Geometry check sheet. Reference: the model listing, model coordinates, mm. Face numbers are marked on the shaded views. A direction names the side the tool comes from. Give positions to 0.01 mm unless a question says otherwise; leave off trailing zeros. Loops run counter-clockwise (first coordinate to the right, second up) from the corner with the lowest first, then second, coordinate; pieces in that order, holes last.
Autodesk Inventor part; units mm, degrees
ref_plane "YZ Plane" through (0, 0, 0) normal (1, 0, 0) x (0, 1, 0)
ref_plane "XZ Plane" through (0, 0, 0) normal (0, 1, 0) x (-1, 0, 0)
ref_plane "XY Plane" through (0, 0, 0) normal (0, 0, 1) x (1, 0, 0)
sketch "Sketch1" plane through (0, 0, 0) normal (0, 0, 1) x (1, 0, 0)
  circle A0 centre (-54.61, 0) radius 11.5 construction
  circle A1 centre (-66.11, 11.5) radius 1.3 construction
  circle A2 centre (-43.11, 11.5) radius 1.3 construction
  circle A3 centre (-66.11, -11.5) radius 1.3 construction
  circle A4 centre (-43.11, -11.5) radius 1.3 construction
  line L0 (-64.77, 10.16) -> (-44.45, 10.16)
  line L1 (-44.45, 10.16) -> (-44.45, -10.16)
  line L2 (-44.45, -10.16) -> (-64.77, -10.16)
  line L3 (-64.77, -10.16) -> (-64.77, 10.16)
  line L4 (-64.77, 10.16) -> (-44.45, -10.16) construction
  line L5 (-44.45, 10.16) -> (-64.77, -10.16) construction
  circle A5 centre (-54.61, 0) radius 7.495
  point P0 (0, 0)
  dimension "d0" = 20.32
  dimension "d1" = 20.32
  dimension "d2" = 14.99
extrude "Extrusion1" add sketch "Sketch1" along normal blind 28 contours L0 L1 L2 L3 | A5
sketch "Sketch2" plane through (0, 0, 0) normal (0, 0, -1) x (-1, 0, 0)
  point P0 (0, 0)
  point P1 (66.11, -11.5)
  point P2 (43.11, -11.5)
  point P3 (43.11, 11.5)
  point P4 (66.11, 11.5)
hole "Hole1" at (-66.11, -11.5, 0) at (-43.11, -11.5, 0) at (-43.11, 11.5, 0) at (-66.11, 11.5, 0) direction (0, 0, 1) diameter 3 depth 8 tip angle 118
sketch "Sketch3" plane through (0, 0, 0) normal (0, 0, -1) x (-1, 0, 0)
  circle A0 centre (54.61, 0) radius 7.495
  circle A1 centre (54.61, 0) radius 2
  point P0 (0, 0)
  dimension "d14" = 4
extrude "Extrusion2" add sketch "Sketch3" along normal blind 1.5 contours A0 | A1
extrude "Extrusion3" add sketch "Sketch3" along normal blind 15 contours A1
chamfer "Chamfer1" distance 0.6 angle 45 1 edges at (-52.61, 0, -15)
fillet "Fillet1" radius 2.16 4 edges at (-64.77, -10.16, 14) (-64.77, 10.16, 14) (-44.45, -10.16, 14) (-44.45, 10.16, 14)
properties part number "Nema 8"
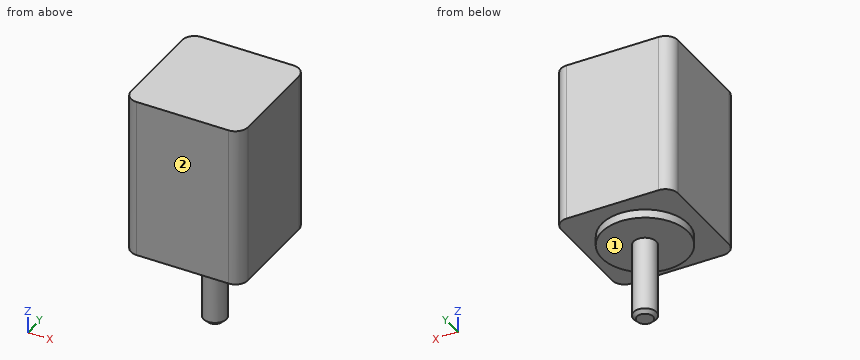
1) Sectioned sample at A-A on y = 0. Enter the section's corners in (x, z) (3 decimals).
2) Sectioned sample at D-D on y = -3.5. Enter the section's corners in (x, z), plus the area to 3 significant figures.
3) Tool access check on the marked faces 1 and 2. Record the directions out of +Z, -Z, +X, -X, +Y, -Y that give a thin tool (end or side, any length) a straight path to the whole face; none if there is none.
4) Depth check by flat-ended pin: P1, Ø2, axis at x = -62.5, y = -2.5, coming from the -Z side; P2, Ø6, axis at y = 1, z = -7.5, coming from the -X side. Enter the tip coordinate at first touch or a pass-through.
5) Sectioned sample at C-C on z = -4. Enter the section's corners in (x, y), plus the area to 3 significant figures.
6) Sectioned sample at B-B on x = -54.61. Enter the section's corners in (y, z) (3 decimals).
7) Scan lines: line 1 along Z through (x, y) = (-58.5, -8.5); line 2 along Z through (x, y) = (-58.25, 5.25); line 3 along X through (y, z) = (9.25, 0.5). Record each from-to range of solid material in increasing order.
Determined:
1. outline: (-64.77, 0) - (-62.105, 0) - (-62.105, -1.5) - (-56.61, -1.5) - (-56.61, -14.4) - (-56.01, -15) - (-53.21, -15) - (-52.61, -14.4) - (-52.61, -1.5) - (-47.115, -1.5) - (-47.115, 0) - (-44.45, 0) - (-44.45, 28) - (-64.77, 28) - close
2. outline: (-64.77, 0) - (-61.24, 0) - (-61.24, -1.5) - (-47.98, -1.5) - (-47.98, 0) - (-44.45, 0) - (-44.45, 28) - (-64.77, 28) - close
2. area: 589 mm2
3. face 1: -Z
3. face 2: +Z, -Z, +X, -X, -Y
4. P1: stops at z = -1.5
4. P2: stops at x = -56.61
5. outline: circle Ø4 at (-54.61, 0)
5. area: 12.6 mm2
6. outline: (-10.16, 0) - (-7.495, 0) - (-7.495, -1.5) - (-2, -1.5) - (-2, -14.4) - (-1.4, -15) - (1.4, -15) - (2, -14.4) - (2, -1.5) - (7.495, -1.5) - (7.495, 0) - (10.16, 0) - (10.16, 28) - (-10.16, 28) - close
7. line 1: z = 0 to 28
7. line 2: z = -1.5 to 28
7. line 3: x = -64.37 to -44.85
